Part model, mm, in its own coordinate system. Face numbers are marked on the shaded views. A direction names the side the tool comes from. Give positions to 0.01 mm unless a question says otherwise; leave off trailing zeros. Write each loop counter-clockwise with the first axis right and the second up, starting at its lowest first coordinate (ties: lowest second). Pieces come first, ordered by that corner, then holes. Notation, with made-up numbers: M -13,-34.75 L 10,-34.75 A24 ccw 10,-10.75 Z; hole C 56.5,15 d5. An arc over 180 degrees is marked long. Answer as CSV lines item,"result". Start each with the question number.
Item 1: Band-saw the part on A-A, the plane y = 0. List the corners of the cut face in (x, z), then the cut area to 3 significant figures.
Item 2: Band-saw the part on C-C, the plane z = 54.5. List the corners of the cut face in (x, y), then the cut area to 3 significant figures.
Item 3: 3-axis set-ups, long thin cutter, end or side, ignore diameter. For the marked faces 1, 2 and 3: which of +Z, -Z, +X, -X, +Y, -Y reach the whole face in a straight line?
Item 4: Wall check: L1, parallel to Z at x = -9.75, y = 0; L2, parallel to X at y = -24, z = 41.5; L3, parallel to X at y = 8, z = 4. Give the ranges that are in metal, low to high. Write a range as from..to.
Item 5: Pin check, flat tips, straight feed: pin 1 (9 mm diameter, centred on y = -2, z = 39.5, fed in from -X); pin 2 (6 mm diameter, centred on x = -102, y = 17.5, fed in from +Z); pin 3 (5 mm diameter, centred on x = -19, y = 13.5, fed in from +Z). Stop position of each tip, or through.
Item 6: Band-saw the part on D-D, the plane z = 15. List the corners of the cut face in (x, y).
Item 7: Band-saw the part on B-B, the plane y = 28. List the corners of the cut face in (x, z).
Item 8: Two-plate mould, pull along X, no slides. Class the marked faces 4, 5 and 6: +X half, -X half, draft (parallel to the pull), parting line (faces both ways), or undercut.
Solid Edge part; units mm, degrees
sketch "Sketch1" plane through (0, 0, 0) normal (1, 0, 0) x (0, 1, 0)
  arc A0 (35, 50) -> (-35, 50) centre (0, 50) ccw
  line L0 (-35, 50) -> (-35, 0)
  line L1 (-35, 0) -> (-10, 0)
  line L2 (-10, 0) -> (-10, 10)
  line L3 (-10, 10) -> (-20, 10)
  line L4 (-20, 10) -> (-20, 20)
  line L5 (-20, 20) -> (0, 20)
  line L6 (0, 20) -> (20, 20)
  line L7 (20, 20) -> (20, 10)
  line L8 (20, 10) -> (10, 10)
  line L9 (10, 10) -> (10, 0)
  line L10 (10, 0) -> (35, 0)
  line L11 (35, 0) -> (35, 50)
extrude "Protrusion1" add sketch "Sketch1" against normal blind 30
sketch "Sketch2" plane through (0, 0, 0) normal (1, 0, 0) x (0, 1, 0)
  circle A0 centre (0, 50) radius 10
extrude "ExtrudedCutout_1" cut sketch "Sketch2" against normal blind 30
sketch "Sketch3" plane through (-30, 0, 42.5) normal (1, 0, 0) x (0, 1, 0)
  line L0 (35, -12.5) -> (-35, -12.5)
  line L1 (-35, -12.5) -> (-35, -42.5)
  line L2 (-35, -42.5) -> (35, -42.5)
  line L3 (35, -42.5) -> (35, -12.5)
extrude "ExtrudedProtrusion_2" add sketch "Sketch3" against normal blind 91.6
sketch "Sketch4" plane through (-121.6, 0, 42.5) normal (1, 0, 0) x (0, 1, 0)
  line L0 (35, 27.5) -> (-35, 27.5)
  line L1 (-35, 27.5) -> (-35, -42.5)
  line L2 (-35, -42.5) -> (35, -42.5)
  line L3 (35, -42.5) -> (35, 27.5)
extrude "ExtrudedProtrusion_3" add sketch "Sketch4" against normal blind 40
sketch "Sketch5" plane through (-80.8, -35, 35) normal (0, -1, 0) x (1, 0, 0)
  circle A0 centre (-80.8, 35) radius 22
extrude "ExtrudedCutout_2" cut sketch "Sketch5" against normal blind 100
sketch "Sketch6" plane through (-121.6, 0, 42.5) normal (1, 0, 0) x (0, 1, 0)
  line L0 (35, -12.5) -> (-35, -12.5)
  line L1 (-35, -12.5) -> (-35, -42.5)
  line L2 (-35, -42.5) -> (35, -42.5)
  line L3 (35, -42.5) -> (35, -12.5)
extrude "ExtrudedProtrusion_4" add sketch "Sketch6" against normal blind 60
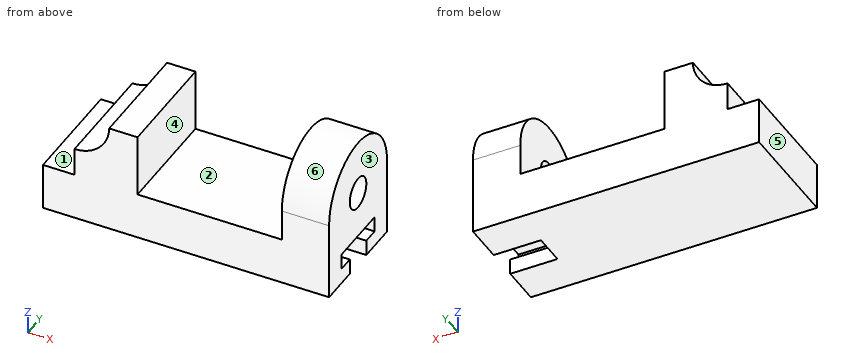
Output:
1,outline,"M -181.6,0 L -30,0 L -30,20 L 0,20 L 0,40 L -30,40 L -30,30 L -121.6,30 L -121.6,70 L -139.6,70 A22 cw -161.6,48 L -161.6,30 L -181.6,30 Z; M -30,60 L 0,60 L 0,85 L -30,85 Z"
1,area,"7,120 mm²"
2,outline,"M -145.99,-35 L -121.6,-35 L -121.6,35 L -145.99,35 Z; M -30,-34.71 L 0,-34.71 L 0,-8.93 L -30,-8.93 Z; M -30,8.93 L 0,8.93 L 0,34.71 L -30,34.71 Z"
2,area,"3,250 mm²"
3,face 1,"+Z, -X, +Y, -Y"
3,face 2,"+Z, +Y, -Y"
3,face 3,"+Z, -Z, +X, +Y, -Y"
4,L1,"20..40, 60..85"
4,L2,"-161.6..-121.6, -30..0"
4,L3,"-181.6..-30"
5,pin 1,"x = -161.6"
5,pin 2,"z = 30"
5,pin 3,"z = 83.23"
6,outline,"M -181.6,-35 L 0,-35 L 0,-20 L -30,-20 L -30,20 L 0,20 L 0,35 L -181.6,35 Z"
7,outline,"M -181.6,0 L 0,0 L 0,71 L -30,71 L -30,30 L -121.6,30 L -121.6,70 L -139.6,70 A22 cw -161.6,48 L -161.6,30 L -181.6,30 Z"
8,face 4,"undercut"
8,face 5,"-X half"
8,face 6,"draft"
